Geometry: see drawing. Coordinates: mm, zero at the bounding-box minimum. Coordinates: 2 decimals unless noted, no trailing zeros. Loops run counter-clockwise (first coordinate to the right, second up) from the corner with the lowest first, then second, coordinate; pieces in that order, holes last. Notation, with made-up numbers: (-36, 65.25) - (-32, 65.25) arc R17 cw to (-32, 92.25) - close; hole circle Ø11 at (14, -26.75). An arc over 180 degrees is marked (long way). Write item = value, one per line. Start each with the question number.
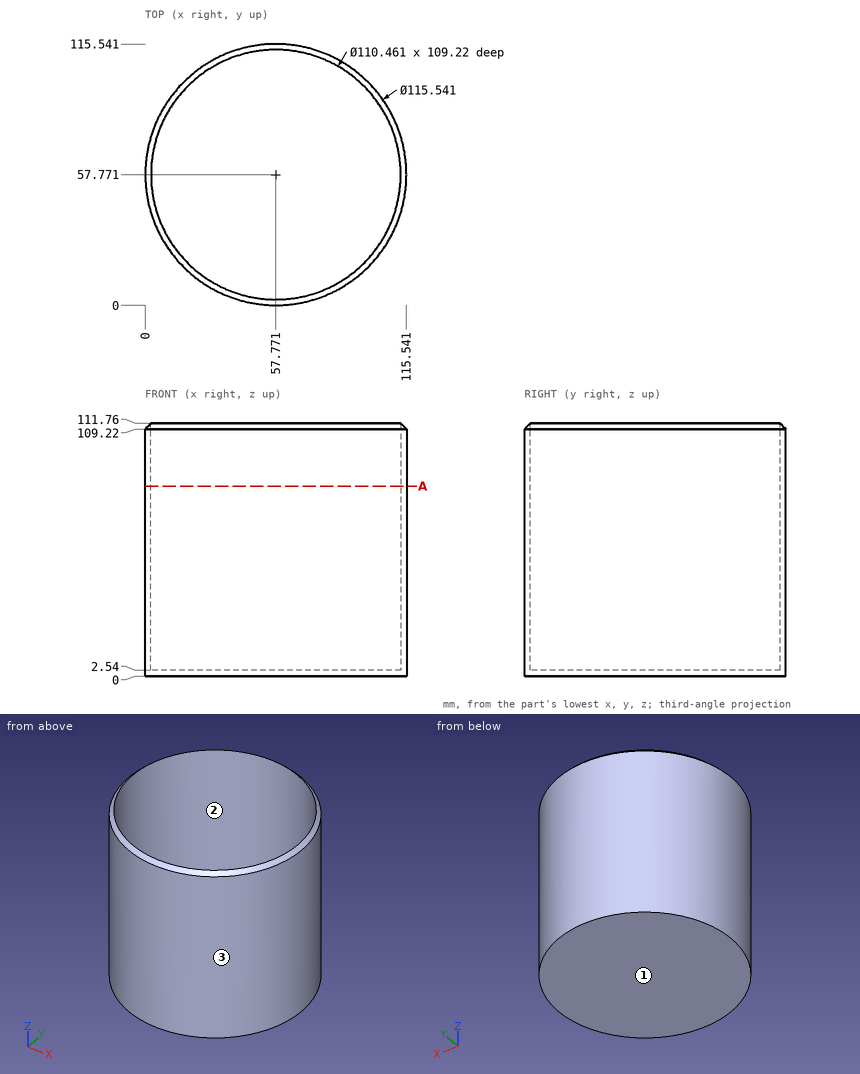
Item 1: Cut plane A-A (z = 84). Return the cut outline in (x, y).
Item 2: First-contact query: pin 1 (5 mm diameter, centred on x = 28.5, z = 41.5, fed in from +Y) (1 decimal); pin 2 (3 mm diameter, centred on y = 45, z = 69, fed in from +X); pin 3 (10 mm diameter, centred on y = 80.5, z = 97, fed in from -X). Flat tips, straight axial feed; report the tip coordinate or a pass-through.
Item 3: Draft query along Y for the marked faces 1, 2 and 3. Return one class per face: released by +Y, released by -Y, zero draft, split by the parting line, or undercut.
Item 4: Material intervals for L1, parallel to X at y = 56, z = 87.5 (1 decimal); L2, parallel to Z at x = 39, y = 89; L3, parallel to Y at x = 73, z = 39.5, sorted ascending. Write a range as [from, to].
Responses:
q1.outline = circle Ø115.54 at (57.77, 57.77); hole circle Ø110.46 at (57.77, 57.77)
q2.pin_1 = 109
q2.pin_2 = 114.43
q2.pin_3 = 2.79
q3.face_1 = zero draft
q3.face_2 = undercut
q3.face_3 = split by the parting line
q4.L1 = [0, 2.6], [113, 115.5]
q4.L2 = [0, 2.54]
q4.L3 = [2.04, 4.68], [110.86, 113.5]
